from build123d import *

# Parameters (mm, degrees)
SKETCH_1_R          = 9
EXTRUDE_3_DEPTH     = 2
SKETCH_2_R          = 1
CUT_EXTRUDE_1_DEPTH = 2
CUT_EXTRUDE_2_DEPTH = 4
SKETCH_6_W          = 1.51058073
SKETCH_6_H          = 3.6
EXTRUDE_4_DEPTH     = 2
CUT_EXTRUDE_3_DEPTH = 2


with BuildPart() as part:
    # 草图1 → 凸台-拉伸3 (new body)
    with BuildSketch(Plane(origin=(0, 0, 0), x_dir=(1, 0, 0), z_dir=(0, 1, 0))):
        with Locations(Location((0, 0, 0), (0, 0, 270))):
            Circle(SKETCH_1_R)
        with BuildLine():
            ThreePointArc((1.526302722, -1.8), (2.36, 0), (1.526302722, 1.8))
            Line((1.526302722, 1.8), (-1.526302722, 1.8))
            ThreePointArc((-1.526302722, 1.8), (-2.36, 0), (-1.526302722, -1.8))
            Line((-1.526302722, -1.8), (1.526302722, -1.8))
        make_face(mode=Mode.SUBTRACT)
    extrude(amount=EXTRUDE_3_DEPTH)

    # 草图2 → 切除-拉伸1 (cut)
    with BuildSketch(Plane(origin=(0, 2, 0), x_dir=(1, 0, 0), z_dir=(0, 1, 0))):
        with Locations(Location((0, 5.8, 0), (0, 0, 270))):
            Circle(SKETCH_2_R)
        with Locations(Location((0, -5.8, 0), (0, 0, 90))):
            Circle(SKETCH_2_R)
    extrude(amount=-CUT_EXTRUDE_1_DEPTH, mode=Mode.SUBTRACT)

    # 草图3 → 切除-旋转1 (revolve, cut)
    with BuildSketch(Plane.XY, mode=Mode.PRIVATE) as cut_revolve_1_sk:
        Polygon((9, 1.526508216), (8.095229941, 1.526508216), (7.409057175, 1.526508216), (7.409057175, 0.419519155), (8.095229941, 0.419519155), (9, 0.419519155), align=None)
    revolve(cut_revolve_1_sk.sketch.rotate(Axis((0, 0, 0), (0, 1, 0)), 90), axis=Axis((0, 0, 0), (0, 1, 0)), mode=Mode.SUBTRACT)

    # 草图4 → 切除-拉伸2 (cut)
    with BuildSketch(Plane(origin=(0, 0, 0), x_dir=(1, 0, 0), z_dir=(0, 1, 0))):
        Polygon((8.707482993, 5.224489796), (5.925925926, 5.224489796), (4.547241119, 5.224489796), (4.547241119, -5.224489796), (5.925925926, -5.224489796), (8.707482993, -5.224489796), (10.594104308, -5.224489796), (10.594104308, 5.224489796), align=None)
    extrude(amount=CUT_EXTRUDE_2_DEPTH, mode=Mode.SUBTRACT)

    # 草图6 → 凸台-拉伸4 (add)
    with BuildSketch(Plane(origin=(0, 2, 0), x_dir=(1, 0, 0), z_dir=(0, 1, 0))):
        with Locations((-2.281593087, 0)):
            Rectangle(SKETCH_6_W, SKETCH_6_H)
        with Locations((2.281593087, 0)):
            Rectangle(SKETCH_6_W, SKETCH_6_H)
    extrude(amount=-EXTRUDE_4_DEPTH)

    # 草图5 → 切除-拉伸3 (cut)
    with BuildSketch(Plane(origin=(0, 2, 0), x_dir=(1, 0, 0), z_dir=(0, 1, 0))):
        with BuildLine():
            Line((1.526302722, 1.8), (1.526302722, -1.8))
            ThreePointArc((1.526302722, -1.8), (0, -2.36), (-1.526302722, -1.8))
            Line((-1.526302722, -1.8), (-1.526302722, 1.8))
            ThreePointArc((-1.526302722, 1.8), (0, 2.36), (1.526302722, 1.8))
        make_face()
    extrude(amount=-CUT_EXTRUDE_3_DEPTH, mode=Mode.SUBTRACT)


solid = part.part
Work out the finished part from the listing and answer in its coordinate system (mm). A direction names the side the tool comes from. Coordinates: 2 decimals unless noted, no trailing zeros. Write each loop counter-clockwise with the first axis right and the second up, starting at its lowest first coordinate (ties: lowest second). Pieces come first, ordered by that corner, then holes. Notation, with made-up numbers: M 46,39 L 55,39 A9 cw 55,53 Z; hole C 74,-29 d10. An arc over 180 degrees is marked long. Use one line per item in the form item = value. Start each with the question number.
1. Straight lines are drawn through the part: probe 1 along Y at (x, z) = (6.25, -5.75); probe 2 along Z at (x, y) = (-0.25, 0.35); probe 3 along X at (y, z) = (1.3, 5.8). For each, find the intervals that lie inside material, in ascending order. Write a range as from..to.
2. The part is cut by section D-D (z = -2). Give the vertices of the cut face in (x, y), plus the area to 3 significant figures.
3. The part is cut by section C-C (y = 1.2). Give the vertices of the cut face in (x, z).
4. A tool of negligible diameter and unlimited length cuts with its end or side. For faces 4 (the face through (-3, 0, 0)), 5 (the face through (0.02, 1.01, 2.36)), 6 (the face through (4.547, 1, 0)), 7 (the face through (-7.405, 0.965, -0.245)), from which of +Z, -Z, +X, -X, +Y, -Y can it reach the whole face along a straight path? Write none if from no direction.
5. The part is cut by section A-A (x = 0). Give the vertices of the cut face in (y, z), plus the area to 3 significant figures.
6. The part is cut by section B-B (z = 0). Give the vertices of the cut face in (x, y).
7. Each of these flat-tipped pins is pushed along its axis until it touches: P1, Ø1.8, axis at x = 0, z = -5.8, coming from the +Y side; P2, Ø1, axis at x = 5.5, y = 2, coming from the -Z side; P3, Ø0.6, axis at y = 0.5, z = -0.5, coming from the +X side. Where does it stop, or does it pass through?
8. The mould has two halves that part along Z. Classify faces 1 (the face through (-8.994, 1.76, -0.318)), 2 (the face through (-3, 2, 0)), 3 (the face through (-0.02, 1.01, -2.36)): released by +Z, released by -Z, zero draft, split by the parting line, or undercut.
Evaluation:
q1.probe_1 = 0..0.42, 1.53..2
q1.probe_2 = -9..-6.77, -4.83..-2.35, 2.35..4.83, 6.77..9
q1.probe_3 = -4.61..-1, 1..4.61
q2.outline = M -8.77,0 L -1.25,0 L -1.25,2 L -8.77,2 L -8.77,1.53 L -7.13,1.53 L -7.13,0.42 L -8.77,0.42 Z; M 1.25,0 L 4.55,0 L 4.55,2 L 1.25,2 Z
q2.area = 19.8 mm^2
q3.outline = M 4.55,-5.22 L 4.55,5.22 L 5.25,5.22 A7.41 ccw long 5.25,-5.22 Z; hole M -1.53,-1.8 A2.36 ccw 1.53,-1.8 L 1.53,1.8 A2.36 ccw -1.53,1.8 Z; hole C 0,-5.8 d2; hole C 0,5.8 d2
q4.face_4 = +Z, -Z, +X, -X, -Y
q4.face_5 = +Y, -Y
q4.face_6 = +X, +Y, -Y
q4.face_7 = none
q5.outline = M 0,-9 L 0.42,-9 L 0.42,-7.41 L 1.53,-7.41 L 1.53,-9 L 2,-9 L 2,-6.8 L 0,-6.8 Z; M 0,-4.8 L 2,-4.8 L 2,-2.36 L 0,-2.36 Z; M 0,2.36 L 2,2.36 L 2,4.8 L 0,4.8 Z; M 0,6.8 L 2,6.8 L 2,9 L 1.53,9 L 1.53,7.41 L 0.42,7.41 L 0.42,9 L 0,9 Z
q5.area = 15.0 mm^2
q6.outline = M -9,0 L -1.53,0 L -1.53,2 L -9,2 L -9,1.53 L -7.41,1.53 L -7.41,0.42 L -9,0.42 Z; M 1.53,0 L 4.55,0 L 4.55,2 L 1.53,2 Z
q7.P1 = through
q7.P2 = -7.48
q7.P3 = 4.55
q8.face_1 = split by the parting line
q8.face_2 = zero draft
q8.face_3 = undercut
